Check sheet for the modelled part. Datum: model origin and axes. Units: mm. Face numbers are marked on the shaded views. A direction names the side the tool comes from. Give positions to 0.01 mm unless a question says otherwise; leave off trailing zeros. Write each loop counter-clockwise with the first axis right and the second up, starting at its lowest first coordinate (ties: lowest second). Pieces come first, ordered by that corner, then holes. Notation, with made-up numbers: M -18.5,76 L -9.5,76 A20 cw -9.5,102 Z; hole C -22.5,-38 d7. An arc over 180 degrees is marked long. Use CSV: the item, a comma, the result in double quotes. Start each with the question number.
1. Cross-section at D-D, the plane y = 14. Enter the section's corners in (x, z).
2. Access from +Z, -Z, +X, -X, +Y, -Y to the whole of each face (thin tool, end or side, straight path). Record for the marked faces 1 and 2.
3. Mould release check, pull along X, two halves, no side actions. Record for the marked faces 3, 4 and 5: +X half, -X half, draft (parallel to the pull), parting line (faces both ways), or undercut.
4. Cross-section at A-A, the plane z = 7.8. Enter the section's corners in (x, y).
5. Scan lines: line 1 (Y direction, x = 24, z = 7.85); line 2 (X direction, y = 26, z = 6.3); line 3 (Y direction, x = 24, z = 5.8). Record each from-to range of solid material in increasing order.
6. Depth check by flat-ended pin: P1, Ø1, axis at y = 21, z = 10, coming from the -X side; P2, Ø5, axis at x = 13, y = 34.5, coming from the -Z side. Enter the tip coordinate at first touch or a pass-through.
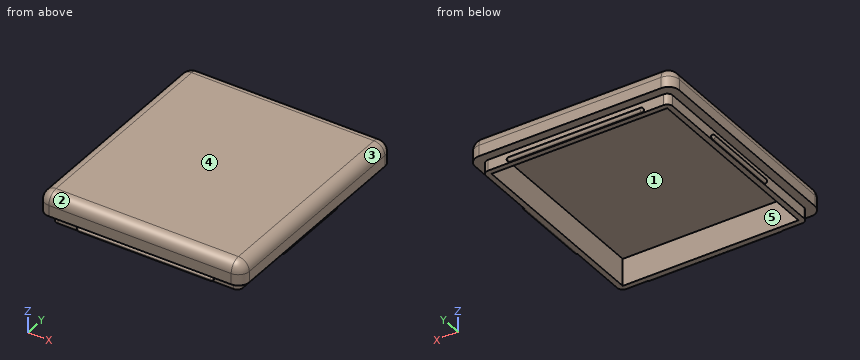
from build123d import *

# Parameters (mm, degrees)
SKETCH043_W     = 37.4
SKETCH043_H     = 41.56
PAD028_DEPTH    = 4
SKETCH044_W     = 34.2
SKETCH044_H     = 38.36
PAD029_DEPTH    = 2
SKETCH045_W     = 32.2
SKETCH045_H     = 36.36
POCKET024_DEPTH = 5
SKETCH046_W     = 25
SKETCH046_H     = 0.8
PAD030_DEPTH    = 0.5
SKETCH047_W     = 15
SKETCH047_H     = 0.8
PAD033_DEPTH    = 0.5
SKETCH054_W     = 15
SKETCH054_H     = 0.8
PAD034_DEPTH    = 0.5
SKETCH055_W     = 25
SKETCH055_H     = 0.8
PAD035_DEPTH    = 0.5
FILLET019_R     = 0.39
FILLET020_R     = 1
FILLET021_R     = 2


with BuildPart() as part:
    # Sketch043 (on DatumPlane) → Pad028 (new body)
    with BuildSketch(Plane.XY.offset(6.7)):
        with Locations((16.9, 22.98)):
            Rectangle(SKETCH043_W, SKETCH043_H)
    extrude(amount=PAD028_DEPTH)

    # Sketch044 (on Face5 of Pad028) → Pad029 (join)
    with BuildSketch(Plane(origin=(0, 0, 6.7), x_dir=(1, 0, 0), z_dir=(0, 0, -1))):
        with Locations((16.9, -22.98)):
            Rectangle(SKETCH044_W, SKETCH044_H)
    extrude(amount=PAD029_DEPTH)

    # Sketch045 (on Face11 of Pad029) → Pocket024 (cut)
    with BuildSketch(Plane(origin=(0, 0, 4.7), x_dir=(1, 0, 0), z_dir=(0, 0, -1))):
        with Locations((16.9, -22.98)):
            Rectangle(SKETCH045_W, SKETCH045_H)
    extrude(amount=-POCKET024_DEPTH, mode=Mode.SUBTRACT)

    # Sketch046 (on Face9 of Pocket024) → Pad030 (join)
    with BuildSketch(Plane(origin=(0, 42.16, 6.7), x_dir=(-1, 0, 0), z_dir=(0, 1, 0))):
        with Locations((-16.9, -1.5)):
            Rectangle(SKETCH046_W, SKETCH046_H)
    extrude(amount=PAD030_DEPTH)

    # Sketch047 (on Face10 of Pad030) → Pad033 (join)
    with BuildSketch(Plane(origin=(-0.2, 0, 6.7), x_dir=(0, -1, 0), z_dir=(-1, 0, 0))):
        with Locations((-23, -1.5)):
            Rectangle(SKETCH047_W, SKETCH047_H)
    extrude(amount=PAD033_DEPTH)

    # Sketch054 (on Face8 of Pad033) → Pad034 (join)
    with BuildSketch(Plane(origin=(34, 0, 6.7), x_dir=(0, 1, 0), z_dir=(1, 0, 0))):
        with Locations((23.01, -1.5)):
            Rectangle(SKETCH054_W, SKETCH054_H)
    extrude(amount=PAD034_DEPTH)

    # Sketch055 (on Face7 of Pad034) → Pad035 (join)
    with BuildSketch(Plane(origin=(0, 3.8, 6.7), x_dir=(1, 0, 0), z_dir=(0, -1, 0))):
        with Locations((16.9, -1.5)):
            Rectangle(SKETCH055_W, SKETCH055_H)
    extrude(amount=PAD035_DEPTH)

    # Fillet019
    fillet019_edges = [part.edges().sort_by_distance(p)[0] for p in [
        (34.5, 23.01, 4.8),
        (34.5, 30.51, 5.2),
        (34.5, 23.01, 5.6),
        (34.25, 30.51, 4.8),
        (34.25, 15.51, 4.8),
        (34.5, 15.51, 5.2),
        (34.25, 15.51, 5.6),
        (34.25, 30.51, 5.6),
        (29.4, 3.55, 5.6),
        (29.4, 3.55, 4.8),
        (29.4, 3.3, 5.2),
        (16.9, 3.3, 4.8),
        (16.9, 3.3, 5.6),
        (4.4, 3.55, 5.6),
        (4.4, 3.55, 4.8),
        (4.4, 3.3, 5.2),
        (-0.45, 15.5, 5.6),
        (-0.45, 15.5, 4.8),
        (-0.7, 15.5, 5.2),
        (-0.7, 23, 4.8),
        (-0.7, 23, 5.6),
        (-0.7, 30.5, 5.2),
        (-0.45, 30.5, 5.6),
        (-0.45, 30.5, 4.8),
        (4.4, 42.41, 5.6),
        (4.4, 42.41, 4.8),
        (4.4, 42.66, 5.2),
        (16.9, 42.66, 4.8),
        (16.9, 42.66, 5.6),
        (29.4, 42.41, 5.6),
        (29.4, 42.66, 5.2),
        (29.4, 42.41, 4.8),
    ]]
    fillet(fillet019_edges, radius=FILLET019_R)

    # Fillet020
    fillet020_edges = [part.edges().sort_by_distance(p)[0] for p in [
        (-0.2, 42.16, 5.7),
        (34, 42.16, 5.7),
        (34, 3.8, 5.7),
        (-0.2, 3.8, 5.7),
    ]]
    fillet(fillet020_edges, radius=FILLET020_R)

    # Fillet021
    fillet021_edges = [part.edges().sort_by_distance(p)[0] for p in [
        (35.6, 2.2, 8.7),
        (16.9, 2.2, 10.7),
        (35.6, 22.98, 10.7),
        (-1.8, 2.2, 8.7),
        (-1.8, 22.98, 10.7),
        (16.9, 43.76, 10.7),
        (35.6, 43.76, 8.7),
        (-1.8, 43.76, 8.7),
    ]]
    fillet(fillet021_edges, radius=FILLET021_R)


solid = part.part
Worked answers:
1,outline,"M -1.8,6.7 L -0.2,6.7 L -0.2,4.7 L 0.8,4.7 L 0.8,9.7 L 33,9.7 L 33,4.7 L 34,4.7 L 34,6.7 L 35.6,6.7 L 35.6,8.7 A2 ccw 33.6,10.7 L 0.2,10.7 A2 ccw -1.8,8.7 Z"
2,face 1,"-Z"
2,face 2,"+Z, +X, -X, -Y"
3,face 3,"+X half"
3,face 4,"draft"
3,face 5,"undercut"
4,outline,"M -1.8,4.2 A2 ccw 0.2,2.2 L 33.6,2.2 A2 ccw 35.6,4.2 L 35.6,41.76 A2 ccw 33.6,43.76 L 0.2,43.76 A2 ccw -1.8,41.76 Z; hole M 0.8,4.8 L 33,4.8 L 33,41.16 L 0.8,41.16 Z"
5,line 1,"y = 2.2 to 4.8, 41.16 to 43.76"
5,line 2,"x = -0.2 to 0.8, 33 to 34"
5,line 3,"y = 3.8 to 4.8, 41.16 to 42.16"
6,P1,"stops at x = -1.63"
6,P2,"stops at z = 9.7"
